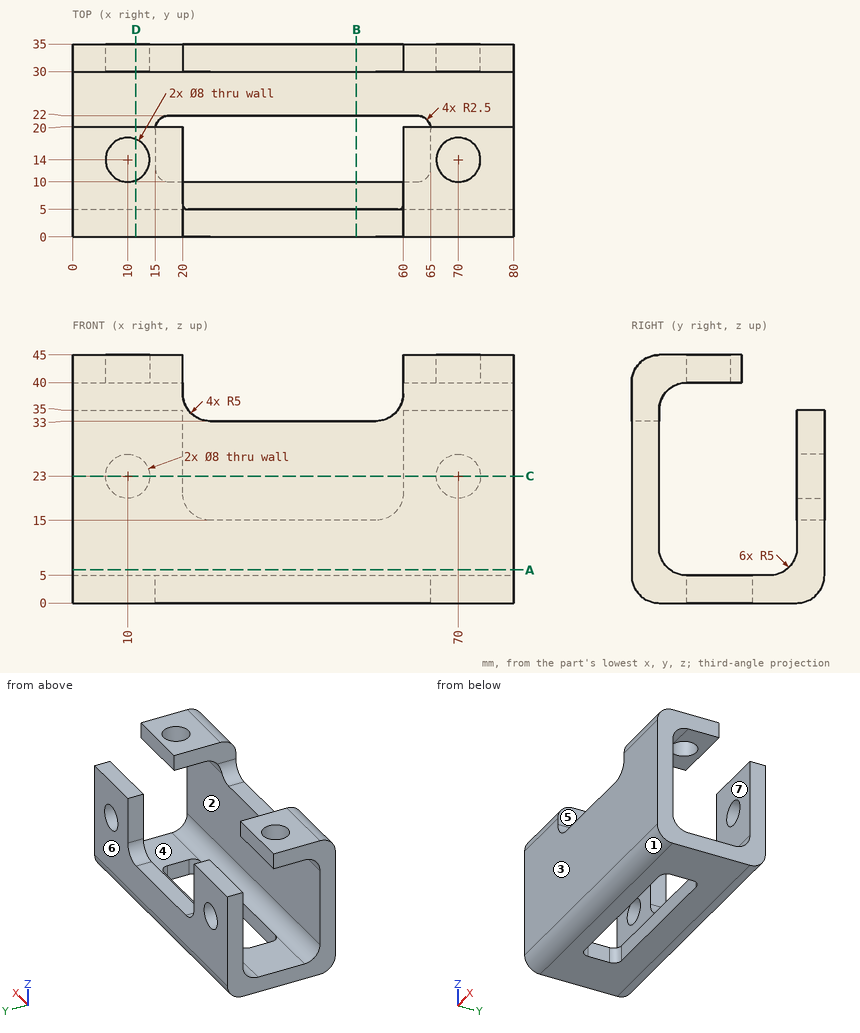
The drawing under review shows one solid part. Ordinate dimensions are in mm from its lowest x, y, z. A direction names the side the tool comes from. Give positions to 0.01 mm unless a question says otherwise; leave off trailing zeros. Write each loop counter-clockwise with the first axis right and the second up, starting at its lowest first coordinate (ties: lowest second). Pieces come first, ordered by that corner, then holes. Notation, with made-up numbers: (63, 11) -> (95, 11) arc R31 cw to (95, 35) -> close; hole circle Ø10 at (23.25, 45). An arc over 180 degrees is marked (long way). Use CSV: the item, a comma, the result in double quotes.
Q1. To check wall thickness, follow probe 1 along X at (y, z) = (33, 23); probe 2 along Y at (x, z) = (51.5, 14); probe 3 along Z at (x, y) = (66.5, 11). State the ranges of each line that lie inside material, in increasing order. Write a range as [from, to].
Conclusion:
probe 1,"[0, 6], [14, 20], [60, 66], [74, 80]"
probe 2,"[0, 5], [30, 35]"
probe 3,"[0, 5], [40, 45]"
Q2. For P1, Ø4, axis at x = 11, y = 31.5, coming from the +Z side; P2, Ø2.5, axis at x = 38.5, z = 3.5, coming from the +Y side; P3, Ø6, axis at x = 55, y = 20, coming from the +Z side; P4, Ø6, axis at x = 28, y = 15.5, coming from the -Z side, all flat-tipped, find the tip position at first contact; note any pin that passes through.
Conclusion:
P1,"z = 35"
P2,"y = 34.99"
P3,"z = 5"
P4,"through"
Q3. Tool access review of the marked faces 4, 5, 6 and 7: name each direction out of +Z, -Z, +X, -X, +Y, -Y from which nothing blocks a thin tool from reaching the whole face with its end or side.
Conclusion:
face 4,"+X, -X"
face 5,"+Z, +Y, -Y"
face 6,"+Z, -Z, +X, -X, +Y"
face 7,"+Z, +X, -X"
Q4. Take a section at B-B, the plane x = 51.5. Write out the cut boundary in (y, z), then the cut area to 3 significant figures.
Conclusion:
outline,"(0, 5) arc R5 ccw to (5, 0) -> (10, 0) -> (10, 5) arc R5 cw to (5, 10) -> (5, 33) -> (0, 33) -> close; (22, 0) -> (30, 0) arc R5 ccw to (35, 5) -> (35, 15) -> (30, 15) -> (30, 10) arc R5 cw to (25, 5) -> (22, 5) -> close"
area,"305 mm2"
Q5. Mouldability with a two-part tool opening along Z and no side actions: class the marked faces 1, 2 and 3 as pulls with the +Z half, pulls with the -Z half, needs draft (parallel to the pull), parting line crosses it, or undercut.
Conclusion:
face 1,"pulls with the -Z half"
face 2,"undercut"
face 3,"needs draft"
Q6. Take a section at A-A, the plane z = 6. Write out the cut boundary in (x, y), then the cut area to 3 significant figures.
Conclusion:
outline,"(0, 0) -> (80, 0) -> (80, 7) -> (0, 7) -> close; (0, 28) -> (80, 28) -> (80, 35) -> (0, 35) -> close"
area,"1,120 mm2"
Q7. Take a section at C-C, the plane z = 23. Write out the cut boundary in (x, y).
Conclusion:
outline,"(0, 0) -> (80, 0) -> (80, 5) -> (0, 5) -> close; (0, 30) -> (6, 30) -> (6, 35) -> (0, 35) -> close; (14, 30) -> (20, 30) -> (20, 35) -> (14, 35) -> close; (60, 30) -> (66, 30) -> (66, 35) -> (60, 35) -> close; (74, 30) -> (80, 30) -> (80, 35) -> (74, 35) -> close"
Q8. Take a section at D-D, the plane x = 11.5. Write out the cut boundary in (y, z), then the cut area to 3 significant figures.
Conclusion:
outline,"(0, 5) arc R5 ccw to (5, 0) -> (30, 0) arc R5 ccw to (35, 5) -> (35, 19.29) -> (30, 19.29) -> (30, 10) arc R5 cw to (25, 5) -> (10, 5) arc R5 cw to (5, 10) -> (5, 35) arc R5 cw to (10, 40) -> (10.29, 40) -> (10.29, 45) -> (5, 45) arc R5 ccw to (0, 40) -> close; (17.71, 40) -> (20, 40) -> (20, 45) -> (17.71, 45) -> close; (30, 26.71) -> (35, 26.71) -> (35, 35) -> (30, 35) -> close"
area,"526 mm2"
